Verification items for the finished model (mm, model axes). A direction names the side the tool comes from. Coordinates: 2 decimals unless noted, no trailing zeros. Order: outer loops, then holes, each group sorted by start corner. A loop starts at its lowest first (then second) coordinate and runs counter-clockwise, first axis right, second up.
Q1. Cross-section at B-B, the plane y = 0. Record the boundary of the cut face in (x, z).
Q2. Depth check by flat-ended pin: P1, Ø1, axis at x = 13.5, z = 12.5, coming from the -Y side; P2, Ø1.8, axis at x = 0, y = 0, coming from the +Z side; P3, Ø8, axis at x = 3, y = 14, coming from the +Z side; P4, Ø4, axis at y = 11.5, z = 6, coming from the +X side. Enter the tip coordinate at first touch or a pass-through.
Q3. Set-up check for faces 1 (the flat face through (2, 28, 10)), 2 (the flat face through (18, 52, 0)), 3 (the flat face through (-10, 27, 2)): record each of +Z, -Z, +X, -X, +Y, -Y from which the full face is reachable in a straight line by a thin tool's end or side.
Q4. Cross-section at A-A, the plane y = 55. Record the boundary of the cut face in (x, z).
Q5. Cross-section at D-D, the plane x = 6.5. Record the boundary of the cut face in (y, z), and give its area (3 significant figures).
Q6. Thickness scan on line 1 (Y direction, x = 0, z = 5); line 2 (X direction, y = 0, z = 5); line 3 (Y direction, x = 20, z = 4). Record the ranges inside material, lowest first.
Q7. Cross-section at C-C, the plane z = 31. Record the boundary of the cut face in (x, y).
Autodesk Inventor part; units mm, degrees
ref_plane "YZ Plane" through (0, 0, 0) normal (1, 0, 0) x (0, 1, 0)
ref_plane "XZ Plane" through (0, 0, 0) normal (0, 1, 0) x (-1, 0, 0)
ref_plane "XY Plane" through (0, 0, 0) normal (0, 0, 1) x (1, 0, 0)
sketch "Sketch9" plane through (0, 0, 0) normal (0, 0, 1) x (1, 0, 0)
  line L0 (0, 0) -> (0, 55) construction
  circle A0 centre (0, 55) radius 1.5
  circle A1 centre (0, 0) radius 1.5
  circle A2 centre (0, 27.5) radius 1.5
  line L1 (-10, 60) -> (10, 60)
  line L2 (10, 60) -> (10, -5)
  line L3 (10, -5) -> (-10, -5)
  line L4 (-10, -5) -> (-10, 60)
  point P0 (-10, 27.5)
  point P1 (0, 60)
  dimension "d35" = 55
  dimension "d36" = 3
  dimension "d37" = 3
  dimension "d38" = 3
  dimension "d39" = 5
  dimension "d40" = 10
extrude "Extrusion9" add sketch "Sketch9" along normal blind 10
sketch "Sketch11" plane through (10, -5, 0) normal (1, 0, 0) x (0, 0, -1)
  line L0 (0, 65) -> (-10, 65)
  line L1 (0, 65) -> (-75, 65)
  line L2 (-75, 65) -> (-75, 50)
  line L3 (-75, 50) -> (0, 50)
  line L4 (0, 50) -> (0, 65)
  point P0 (0, 5)
  dimension "d43" = 15
  dimension "d44" = 75
extrude "Extrusion10" add sketch "Sketch11" along normal blind 35
sketch "Sketch12" plane through (-10, 60, 10) normal (0, 1, 0) x (1, 0, 0)
  line L0 (20, -65) -> (20, 0)
  line L1 (20, -65) -> (34, -65)
  line L2 (34, -65) -> (34, 0)
  line L3 (34, 0) -> (20, 0)
  line L4 (20, 0) -> (20, -65)
  point P0 (10, 10)
  dimension "d47" = 14
extrude "Extrusion11" cut sketch "Sketch12" against normal through all
chamfer "Chamfer6" distance 14 angle 45 1 edges at (24, 52.5, 10)
sketch "Sketch14" plane through (10, 45, 0) normal (0, -1, 0) x (1, 0, 0)
  line L0 (0, 10) -> (14, 24)
  line L1 (15.4558, 0) -> (35, 19.5442)
  line L2 (35, 75) -> (35, 0)
  line L3 (0, 0) -> (35, 0)
  line L4 (15.4558, 0) -> (35, 0)
  line L5 (35, 19.5442) -> (35, 0)
  point P0 (-10, 0)
  dimension "d73" = 18
extrude "Extrusion13" cut sketch "Sketch14" against normal through all
sketch "Sketch15" plane through (0, 0, 0) normal (0, 0, -1) x (-1, 0, 0)
  line L0 (-25.4558, 60) -> (-25.4558, 45)
  line L1 (-10, 45) -> (-25.4558, 45)
  line L2 (-10, 45) -> (-10, -5)
  line L3 (-10, -5) -> (10, -5)
  line L4 (10, -5) -> (10, 60)
  line L5 (10, 60) -> (-25.4558, 60)
  circle A0 centre (0, 55) radius 1.5
  circle A1 centre (0, 0) radius 1.5
  circle A2 centre (0, 27.5) radius 1.5
  line L6 (-10, -5) -> (10, -5)
  line L7 (10, 60) -> (-10, 60)
  line L8 (-10, -5) -> (-10, 60)
  line L9 (-10, 60) -> (10, 60)
extrude "Extrusion14" add sketch "Sketch15" along normal blind 3 contours L5 L4 L3 L2 L8
chamfer "Chamfer8" distance 3 angle 45 1 edges at (-10, 27.5, 10)
sketch "Sketch17" plane through (-10, -5, -3) normal (0, -1, 0) x (1, 0, 0)
  line L0 (20, 3) -> (20, 13)
  line L1 (20, 3) -> (35.4558, 3)
  line L2 (20, 3) -> (35.4558, 3)
  line L3 (35.4558, 3) -> (37.5981, 4.5)
  line L4 (37.5981, 4.5) -> (49, 4.5)
  line L5 (49, 6.5) -> (36.9675, 6.5)
  line L6 (36.9675, 6.5) -> (34.8252, 5)
  line L7 (34.8252, 5) -> (20, 5)
  line L8 (20, 3) -> (20, 5)
  line L9 (49, 6.5) -> (49, 4.5)
  point P0 (10, 3)
  point P1 (55, 22.5442)
  dimension "d83" = 215
  dimension "d84" = 2
  dimension "d88" = 1.5
  dimension "d89" = 6
extrude "Extrusion16" add sketch "Sketch17" against normal blind 65
sketch "Sketch18" plane through (24, 60, 75) normal (0, 1, 0) x (1, 0, 0)
  line L0 (15, 73.5) -> (3.5981, 73.5)
  line L1 (4.9558, 71.5) -> (15, 71.5)
  line L2 (15, 71.5) -> (15, 73.5)
  line L3 (3.5981, 73.5) -> (4.9558, 71.5)
  point P0 (-24, 75)
extrude "Extrusion17" cut sketch "Sketch18" against normal through all
sketch "Sketch19" plane through (-10, -5, -3) normal (0, -1, 0) x (1, 0, 0)
  line L0 (34.8252, 5) -> (20, 5)
  line L1 (20, 3) -> (35.4558, 3)
  line L2 (35.4558, 3) -> (37.5981, 4.5)
  line L3 (37.5981, 4.5) -> (38.9558, 6.5)
  line L4 (38.9558, 6.5) -> (36.9675, 6.5)
  line L5 (36.9675, 6.5) -> (34.8252, 5)
  line L6 (20, 3) -> (20, 5)
  point P0 (10, 3)
extrude "Extrusion18" cut sketch "Sketch19" against normal blind 50
equation "\"Module\" = 2"
equation "\"PressureAngle\" = 20deg"
equation "\"UnitProfileClearance\" = 0.25"
equation "\"UnitRoundRadius\" = 0.35"
equation "\"HeadDiameter\" = 42"
equation "\"RootDiameter\" = 33"
equation "\"BaseDiameter\" = 35.70832"
equation "\"PitchDiameter\" = 38"
equation "\"HelixAngle\" = 0"
equation "\"UnitCorrection\" = 0"
equation "\"UnitAddendumModification\" = 0"
equation "\"CircularPitch\" = 6.283185"
equation "\"UnitBacklashShift\" = 0"
equation "\"TotalToolShift\" = 0"
equation "\"IsInternal\" = 0"
properties part number "GA04" material "ABS Plastic"
Check values:
1. outline: (-10, -3) - (-1.5, -3) - (-1.5, 10) - (-7, 10) - (-10, 7) - close; (1.5, -3) - (10, -3) - (10, 10) - (1.5, 10) - close
2. P1: stops at y = 45
2. P2: passes through
2. P3: stops at z = 10
2. P4: stops at x = 10
3. face 1: +Z, -X, +Y, -Y
3. face 2: -Z, +X, +Y, -Y
3. face 3: +Z, -Z, -X, +Y, -Y
4. outline: (-10, -3) - (-1.5, -3) - (-1.5, 10) - (-7, 10) - (-10, 7) - close; (1.5, -3) - (10, -3) - (10, 0) - (25.46, 0) - (27.6, 1.5) - (28.96, 3.5) - (45, 19.54) - (45, 75) - (24, 75) - (24, 24) - (10, 10) - (1.5, 10) - close
5. outline: (-5, -3) - (60, -3) - (60, 10) - (-5, 10) - close
5. area: 845 mm2
6. line 1: y = -5 to -1.5, 1.5 to 26, 29 to 53.5, 56.5 to 60
6. line 2: x = -10 to -1.5, 1.5 to 10
6. line 3: y = 45 to 60
7. outline: (24, 45) - (45, 45) - (45, 60) - (24, 60) - close
